```python
from build123d import *

# Parameters (mm, degrees)
SKETCH_1_W                                = 375
SKETCH_1_H                                = 375
EXTRUDE_1_DEPTH                           = 22
CHAMFER_1_SIZE                            = 30
CUT_EXTRUDE_1_DEPTH                       = 267.076116929
MIRROR_1_AT_THE_SECOND_PLANE_COPY_1_DEPTH = 267.076116929
SKETCH_3_R                                = 155
EXTRUDE_2_DEPTH                           = 23
SKETCH_4_R                                = 95
CUT_EXTRUDE_2_DEPTH                       = 3
SKETCH_5_R                                = 15
EXTRUDE_3_DEPTH                           = 15
CUT_EXTRUDE_3_DEPTH                       = 267.85670312
WRAP_1_SECTION_W                          = 0.2
WRAP_1_SECTION_H                          = 9
WRAP_1_ANGLE                              = 0.036965019


with BuildPart() as part:
    # 草图1 → 凸台-拉伸1 (new body)
    with BuildSketch(Plane.XY):
        Rectangle(SKETCH_1_W, SKETCH_1_H)
    extrude(amount=EXTRUDE_1_DEPTH)

    # 倒角1
    chamfer_1_edges = [part.edges().sort_by_distance(p)[0] for p in [
        (187.5, -187.5, 11),
        (-187.5, -187.5, 11),
        (-187.5, 187.5, 11),
        (187.5, 187.5, 11),
    ]]
    chamfer(chamfer_1_edges, length=CHAMFER_1_SIZE)

    # 草图2 → 切除-拉伸1 (cut, through all)
    with BuildSketch(Plane.XY.offset(22)):
        with BuildLine():
            Line((125, -187.5), (125, -165))
            ThreePointArc((125, -165), (135, -155), (145, -165))
            Line((145, -165), (145, -187.5))
            ThreePointArc((145, -187.5), (135, -197.5), (125, -187.5))
        make_face()
    cut_extrude_1 = extrude(amount=-CUT_EXTRUDE_1_DEPTH, mode=Mode.SUBTRACT)

    # 镜向1: 切除-拉伸1 across plane
    add(cut_extrude_1.mirror(Plane.ZX), mode=Mode.SUBTRACT)

    # 镜向1 at the second plane: 切除-拉伸1 across plane
    add(cut_extrude_1.mirror(Plane(origin=(0, 0, 0), x_dir=(0, 0, 1), z_dir=(1, 0, 0))), mode=Mode.SUBTRACT)

    # 镜向1 at the second plane copy 1 sket → 镜向1 at the second plane copy 1 (cut, through all)
    with BuildSketch(Plane(origin=(0, 0, 22), x_dir=(-1, 0, 0), z_dir=(0, 0, 1))):
        with BuildLine():
            Line((125, -187.5), (125, -165))
            ThreePointArc((125, -165), (135, -155), (145, -165))
            Line((145, -165), (145, -187.5))
            ThreePointArc((145, -187.5), (135, -197.5), (125, -187.5))
        make_face()
    extrude(amount=-MIRROR_1_AT_THE_SECOND_PLANE_COPY_1_DEPTH, mode=Mode.SUBTRACT)

    # 草图3 → 凸台-拉伸2 (add)
    with BuildSketch(Plane.XY.offset(22)):
        Circle(SKETCH_3_R)
    extrude(amount=EXTRUDE_2_DEPTH)

    # 草图4 → 切除-拉伸2 (cut)
    with BuildSketch(Plane.XY.offset(45)):
        Circle(SKETCH_4_R)
    extrude(amount=-CUT_EXTRUDE_2_DEPTH, mode=Mode.SUBTRACT)

    # 草图5 → 凸台-拉伸3 (add)
    with BuildSketch(Plane.XY.offset(42)):
        Circle(SKETCH_5_R)
    extrude(amount=EXTRUDE_3_DEPTH)

    # 草图6 → 切除-旋转1 (revolve, cut)
    with BuildSketch(Plane(origin=(0, 0, 0), x_dir=(0, 0, -1), z_dir=(1, 0, 0)), mode=Mode.PRIVATE) as cut_revolve_1_sk:
        Polygon((-78.588457268, -132), (-27, -118.176914536), (-27, -145.823085464), align=None)
    revolve(cut_revolve_1_sk.sketch.rotate(Axis((0, 0, 0), (0, 0, -1)), 270), axis=Axis((0, 0, 0), (0, 0, -1)), mode=Mode.SUBTRACT)

    # 草图7 → 切除-拉伸3 (cut, through all)
    with BuildSketch(Plane.XY.offset(27)):
        with BuildLine():
            Line((-16, 117.088783106), (-16, 144.942651605))
            ThreePointArc((-16, 144.942651605), (0, 145.823085464), (16, 144.942651605))
            Line((16, 144.942651605), (16, 117.088783106))
            ThreePointArc((16, 117.088783106), (0, 118.176914536), (-16, 117.088783106))
        make_face()
    extrude(amount=-CUT_EXTRUDE_3_DEPTH, mode=Mode.SUBTRACT)

    # 包覆1 section (on wrap section) → 包覆1 (revolve, cut)
    with BuildSketch(Plane(origin=(0, 0, 22), x_dir=(0.9999999479708641, 0.00032258063956674645, 0), z_dir=(-0.00032258063956674645, 0.9999999479708641, 0))):
        with Locations((154.9, -18.5)):
            Rectangle(WRAP_1_SECTION_W, WRAP_1_SECTION_H)
    wrap_1 = revolve(axis=Axis((0, 0, 22), (0, 0, -1)), revolution_arc=WRAP_1_ANGLE, mode=Mode.SUBTRACT)

    # 镜向2: 包覆1 across plane
    add(wrap_1.mirror(Plane(origin=(0, 0, 0), x_dir=(0, 0, 1), z_dir=(1, 0, 0))), mode=Mode.SUBTRACT)


solid = part.part
```
Could you check a few things on this model? Use its own coordinates, in mm. A direction names the side the tool comes from. Coordinates: 2 decimals unless noted, no trailing zeros. Write each loop counter-clockwise with the first axis right and the second up, starting at its lowest first coordinate (ties: lowest second). Pieces come first, ordered by that corner, then holes. Notation, with made-up numbers: (24.25, 69.5) -> (52.25, 69.5) arc R13 ccw to (52.25, 89.5) -> close; hole circle Ø11 at (68.25, 8.25). An arc over 180 degrees is marked (long way). Return JSON: item names as keys, results as strings.
(1) Imagine slicing it at B-B, the plane z = 52. Please give me the cut outline in (x, y), then the cut area to 3 significant figures.
Numbers:
{"outline": "circle Ø30 at (0, 0)", "area": "707 mm2"}
(2) I need wall thicknesses on L1, parallel to Y at x = 53, z = 36.5; L2, parallel to Y at x = 0, z = 44.05; L3, parallel to Y at x = 0, z = 43. Which ranges of each line are inside material? Lowest first, please.
Numbers:
{"L1": "y = -145.66 to -133.11, -108.47 to 108.47, 133.11 to 145.66", "L2": "y = -155 to -141.25, -122.75 to -95, -15 to 15, 95 to 122.75, 141.25 to 155", "L3": "y = -155 to -141.54, -122.46 to -95, -15 to 15, 95 to 122.46, 141.54 to 155"}
(3) We'd pull the mould along Z, two halves only. Please class faces 6 (the conical face through (-112.079, 85.939, 44.126)), 7 (the flat face through (-172, -173, 11)), 8 (the flat face through (34, -137, 45)): +Z half, -Z half, draft (parallel to the pull), parting line (faces both ways), or undercut.
Numbers:
{"face 6": "undercut", "face 7": "draft", "face 8": "+Z half"}
(4) I'm going to push flat-ended pins straight in: pin 1 (24 mm diameter, centred on y = 171, z = 7, fed in from -X); pin 2 (17.5 mm diameter, centred on y = -180, z = 11, fed in from -X); pin 3 (10 mm diameter, centred on x = 5.5, y = -48.5, fed in from -Z); pin 4 (2 mm diameter, centred on y = 129, z = 36, fed in from -X). Where does each tip first touch, or does it pass through?
Numbers:
{"pin 1": "stops at x = -186", "pin 2": "stops at x = -173.75", "pin 3": "stops at z = 0", "pin 4": "stops at x = -87.41"}
(5) Imagine slicing it at A-A, the plane x = 0. Please give me the cut outline in (y, z).
Numbers:
{"outline": "(-187.5, 0) -> (118.18, 0) -> (118.18, 27) -> (123, 45) -> (95, 45) -> (95, 42) -> (15, 42) -> (15, 57) -> (-15, 57) -> (-15, 42) -> (-95, 42) -> (-95, 45) -> (-123, 45) -> (-118.18, 27) -> (-145.82, 27) -> (-141, 45) -> (-155, 45) -> (-155, 22) -> (-187.5, 22) -> close; (141, 45) -> (145.82, 27) -> (145.82, 0) -> (187.5, 0) -> (187.5, 22) -> (155, 22) -> (155, 45) -> close"}
(6) Which directions (+Z, -Z, +X, -X, +Y, -Y) give clear straight access to the entire face, cutting with the end or side of a thin tool? Please do faces 1 (the flat face through (-145, 176, 11)), 2 (the flat face through (151, 187.5, 11)), 3 (the cylindrical face through (147.84, 46.56, 33.34)), 4 (the flat face through (145, -176, 11)), 5 (the cylindrical face through (-0.224, 145.823, 13.689)).
Numbers:
{"face 1": "+Z, -Z, +Y", "face 2": "+Z, -Z, +X, -X, +Y", "face 3": "+Z", "face 4": "+Z, -Z, -Y", "face 5": "-Z"}
